Verification items for the finished model (mm, model axes). A direction names the side the tool comes from. Give positions to 0.01 mm unless a question says otherwise; leave off trailing zeros. Order: outer loops, then holes, each group sorted by start corner. A loop starts at its lowest first (then second) coordinate and runs counter-clockwise, first axis right, second up. Notation, with made-up numbers: M -18,-18.5 L 10,-18.5 A32 cw 10,18.5 Z; hole C 83.5,89.25 d8. An arc over 180 degrees is marked long. Answer as a JSON object with one key per item and string values.
```python
from build123d import *

# Parameters (mm, degrees)
F2_R     = 1.5
F4_DEPTH = 25.4
F3_R     = 1.5
F5_DEPTH = 25.4


with BuildPart() as f1:
    # F0 (on Front) → F1 (revolve)
    with BuildSketch(Plane.XZ):
        Polygon((0, 48.046581), (0, 15.846581), (13.95, 15.846581), (13.95, 36.064981), (2.5, 36.046581), (2.5, 48.046581), align=None)
    revolve(axis=Axis((0, 0, 31.946581), (0, 0, -1)))

    # F2 (on Top) → F4 (cut)
    with BuildSketch(Plane.XY):
        with Locations((6.717514, -6.717514)):
            Circle(F2_R)
        with Locations((-6.717514, 6.717514)):
            Circle(F2_R)
    extrude(amount=F4_DEPTH, mode=Mode.SUBTRACT)

    # F3 (on Top) → F5 (cut)
    with BuildSketch(Plane.XY):
        with Locations((-5.656854, -5.656854)):
            Circle(F3_R)
        with Locations((5.656854, 5.656854)):
            Circle(F3_R)
    extrude(amount=F5_DEPTH, mode=Mode.SUBTRACT)


solid = f1.part
```
Q1. Gauge pin test, flat ends, axial feed: pin 1 Ø3 at (y, z) = (-3, 29) entering from +X; pin 2 Ø0.9 at (x, y) = (-6.5, 7) entering from -Z; pin 3 Ø5 at (x, y) = (6.72, -6.72) entering from +Z. Record the tip position at first contact, or that the pin passes through.
Resolved:
{"pin 1": "stops at x = 13.87", "pin 2": "stops at z = 25.4", "pin 3": "stops at z = 36.06"}
Q2. Section check C-C on z = 31.5. Record the cut outline in (x, y), then the cut area to 3 significant figures.
Resolved:
{"outline": "C 0,0 d27.9", "area": "611 mm²"}
Q3. Release check for a two-part mould opening along Y. For faces 1 (the face through (-0.54, 2.44, 42.13)), 2 (the face through (-4.226, -5.206, 20.556)) record: +Y half, -Y half, draft (parallel to the pull), parting line (faces both ways), or undercut.
Resolved:
{"face 1": "parting line", "face 2": "undercut"}
Q4. Section check D-D on z = 39.5. Record the cut outline in (x, y), then the cut area to 3 significant figures.
Resolved:
{"outline": "C 0,0 d5", "area": "19.6 mm²"}
Q5. Material ranges on L1, parallel to Z at x = -5.75, y = -7.75; L2, parallel to X at y = 0.5, z = 28; L3, parallel to X at y = 5.5, z = 31.5, recorded low to high.
Resolved:
{"L1": "z = 15.85 to 36.06", "L2": "x = -13.94 to 13.94", "L3": "x = -12.82 to 12.82"}
Q6. Tool access check on faces 3 (the face through (5.462, 7.144, 20.556)), 4 (the face through (-3.02, 13.62, 26.1)). Record the directions out of +Z, -Z, +X, -X, +Y, -Y that give a thin tool (end or side, any length) a straight path to the whole face; none if there is none.
Resolved:
{"face 3": "-Z", "face 4": "+Z, -Z"}
Q7. Section check A-A on x = 0. Record the cut outline in (y, z).
Resolved:
{"outline": "M -13.95,15.85 L 13.95,15.85 L 13.95,36.06 L 2.5,36.05 L 2.5,48.05 L -2.5,48.05 L -2.5,36.05 L -13.95,36.06 Z"}
